Source: three-view drawing plus pictorial views. Frame: mm from the lowest corner of the part. A direction names the side the tool comes from. Coordinates: 2 decimals unless noted, no trailing zeros. Write each loop counter-clockwise with the first axis right and the second up, starting at its lowest first coordinate (ties: lowest second). Pieces come first, ordered by that corner, then holes. Notation, with made-up numbers: M 57,-19.75 L 90,-19.75 A23 cw 90,5.25 Z; hole C -14,25.25 d4. An arc over 180 degrees is marked long. Write item = value, one per line. Start each with the question number.
Item 1: Reachability of the marked faces 1 and 2 from +Z, -Z, +X, -X, +Y, -Y: full face, straight path, thin tool, end or side. Return the list, or none.
Item 2: Ray query, L1, parallel to Y at x = 0.9, z = 3; L2, parallel to Z at x = 2.4, y = 33; L3, parallel to Y at x = 2.75, z = 3.5. Return the intervals inside material, ascending. Write a range as [from, to].
Item 3: Section B-B on x = 0.5. Output: boundary loops of the cut face in (y, z).
Item 4: Section D-D on y = 25. Output: boundary loops of the cut face in (x, z), plus the area to 3 significant figures.
Item 5: Section A-A on z = 3. Output: boundary loops of the cut face in (x, y).
Item 6: Section C-C on y = 15.4. Output: boundary loops of the cut face in (x, z).
Item 7: First-contact query: pin 1 Ø2 at (y, z) = (3.4, 3) entering from +X; pin 2 Ø0.9 at (x, z) = (1.5, 3) entering from +Y; pin 3 Ø1.5 at (x, y) = (1, 22.5) entering from -Z. Flat tips, straight axial feed; report the tip coordinate or a pass-through.
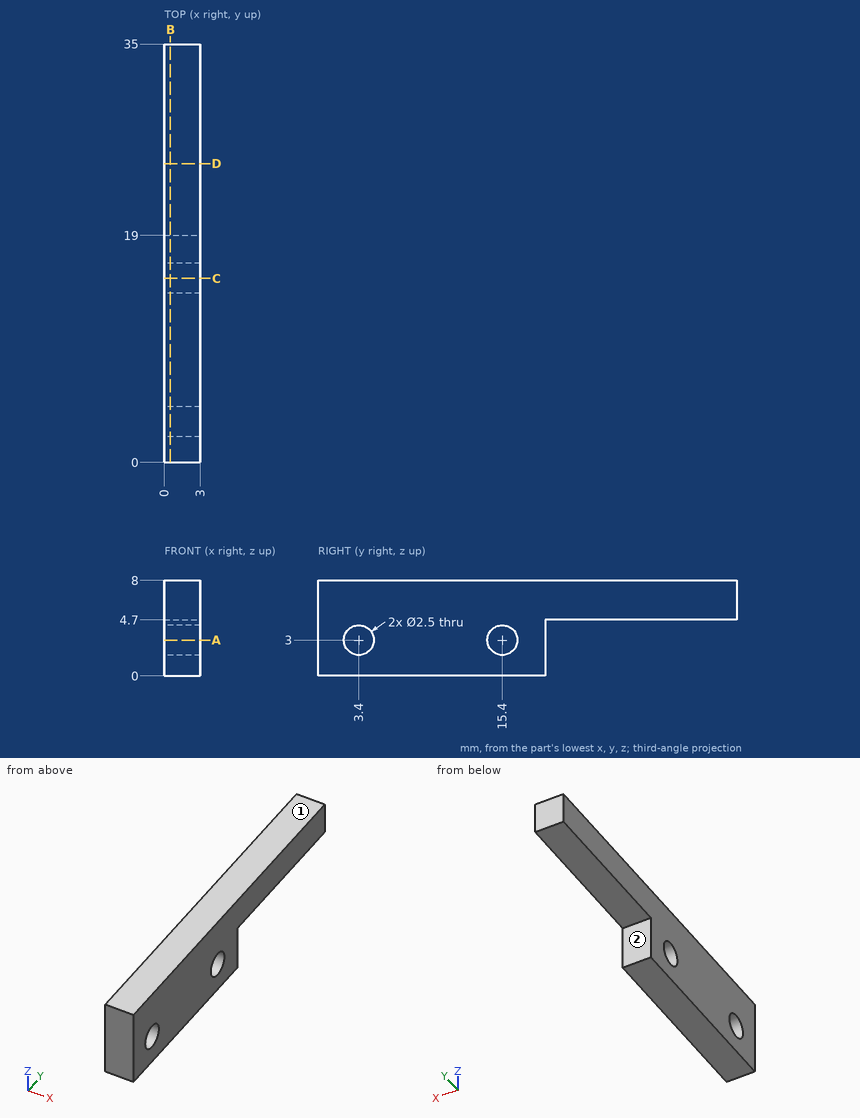
Responses:
q1.face_1 = +Z, +X, -X, +Y, -Y
q1.face_2 = -Z, +X, -X, +Y
q2.L1 = [0, 2.15], [4.65, 14.15], [16.65, 19]
q2.L2 = [4.7, 8]
q2.L3 = [0, 2.25], [4.55, 14.25], [16.55, 19]
q3.outline = M 0,0 L 19,0 L 19,4.7 L 35,4.7 L 35,8 L 0,8 Z; hole C 3.4,3 d2.5; hole C 15.4,3 d2.5
q4.outline = M 0,4.7 L 3,4.7 L 3,8 L 0,8 Z
q4.area = 9.90 mm²
q5.outline = M 0,0 L 3,0 L 3,2.15 L 0,2.15 Z; M 0,4.65 L 3,4.65 L 3,14.15 L 0,14.15 Z; M 0,16.65 L 3,16.65 L 3,19 L 0,19 Z
q6.outline = M 0,0 L 3,0 L 3,1.75 L 0,1.75 Z; M 0,4.25 L 3,4.25 L 3,8 L 0,8 Z
q7.pin_1 = through
q7.pin_2 = 19
q7.pin_3 = 4.7
